Check sheet for the modelled part. Datum: model origin and axes. Units: mm. A direction names the side the tool comes from. Give positions to 0.01 mm unless a question says otherwise; leave off trailing zeros. Order: outer loops, then holes, each group sorted by start corner. A loop starts at its lowest first (then second) coordinate and runs counter-clockwise, first axis right, second up. Notation, with made-up numbers: M -18.75,28.5 L -9.75,28.5 A11 cw -9.75,47.5 Z; hole C -10,12.5 d2. An arc over 180 degrees is marked long. Answer in a Markdown table with one row per item. Add a question column.
from build123d import *

# Parameters (mm, degrees)
SKETCH_1_W      = 20
SKETCH_1_H      = 280
EXTRUDE_1_DEPTH = 100
SKETCH_2_W      = 100
SKETCH_2_H      = 80
EXTRUDE_2_DEPTH = 20


with BuildPart() as part:
    # 草图1 → 凸台-拉伸1 (new body)
    with BuildSketch(Plane.XY):
        Rectangle(SKETCH_1_W, SKETCH_1_H)
    extrude(amount=EXTRUDE_1_DEPTH)

    # 草图2 → 凸台-拉伸2 (add)
    with BuildSketch(Plane.ZY.offset(10)):
        with Locations((150, -100)):
            Rectangle(SKETCH_2_W, SKETCH_2_H)
    extrude(amount=-EXTRUDE_2_DEPTH)


solid = part.part
Q1. Cross-section at B-B (y = -2). Record the boundary of the cut face in (x, z).
Q2. Cross-section at C-C (z = 165). Record the boundary of the cut face in (x, y).
Q3. Tool access check on faces 1 (the flat face through (0, -60, 149)), 2 (the flat face through (0, -140, 99)). Record the directions out of +Z, -Z, +X, -X, +Y, -Y that give a thin tool (end or side, any length) a straight path to the whole face; none if there is none.
Q4. Cross-section at A-A (x = 0.5). Record the boundary of the cut face in (y, z).
Q5. Go/stop test with flat-tipped pins: pin 1 (10 mm diameter, centred on x = 3, y = 59.5, fed in from +Z); pin 2 (1.5 mm diameter, centred on x = -2.5, z = 114, fed in from +Y). Record where each tip stops, or that it passes through.
Q6. Thickness scan on probe 1 along Z at (x, y) = (-2, 42); probe 2 along Y at (x, z) = (-8.75, 169). Record the ranges inside material, lowest first.
Values follow:
| question | item | result |
|---|---|---|
| 1 | outline | M -10,0 L 10,0 L 10,100 L -10,100 Z |
| 2 | outline | M -10,-140 L 10,-140 L 10,-60 L -10,-60 Z |
| 3 | face 1 | +Z, +X, -X, +Y |
| 3 | face 2 | +Z, -Z, +X, -X, -Y |
| 4 | outline | M -140,0 L 140,0 L 140,100 L -60,100 L -60,200 L -140,200 Z |
| 5 | pin 1 | z = 100 |
| 5 | pin 2 | y = -60 |
| 6 | probe 1 | 0 to 100 |
| 6 | probe 2 | -140 to -60 |
